Read the model definition and answer for the solid it produces. Units are mm, in the model's axes. Round coordinates to 2 decimals unless told otherwise and drop trailing zeros. Order: outer loops, then holes, each group sorted by start corner. A loop starts at its lowest first (then second) coordinate and runs counter-clockwise, first axis right, second up.
Autodesk Inventor part; units mm, degrees
ref_plane "YZ Plane" through (0, 0, 0) normal (1, 0, 0) x (0, 1, 0)
ref_plane "XZ Plane" through (0, 0, 0) normal (0, 1, 0) x (-1, 0, 0)
ref_plane "XY Plane" through (0, 0, 0) normal (0, 0, 1) x (1, 0, 0)
sketch "스케치1" plane through (0, 0, 0) normal (0, 1, 0) x (-1, 0, 0)
  circle A0 centre (0, 0) radius 15
  circle A1 centre (0, 0) radius 11.5
  line L0 (-14.5237, 3.75) -> (-45, 3.75)
  line L1 (-45, 3.75) -> (-45, -3.75)
  line L2 (-45, -3.75) -> (-14.5237, -3.75)
  line L3 (-14.5237, -3.75) -> (-14.5237, 3.75)
  dimension "d0" = 30
  dimension "d1" = 23
  dimension "d2" = 7.5
  dimension "d3" = 3.75
  dimension "d4" = 45
extrude "돌출1" add sketch "스케치1" along normal blind 1
properties part number "압력센서"
Q1. A cutting plane is placed at A-A, the plane x = 0. Give the vertices of the cut face in (y, z), plus the area to 3 significant figures.
Outcome:
outline: (0, -15) - (1, -15) - (1, -11.5) - (0, -11.5) - close; (0, 11.5) - (1, 11.5) - (1, 15) - (0, 15) - close
area: 7.00 mm2
Q2. Straight lines are drawn through the part: probe 1 along Z at (x, y) = (0, 0.2); probe 2 along X at (y, z) = (0.65, -3); probe 3 along X at (y, z) = (0.35, 1). For each, find the intervals that lie inside material, in ascending order.
Outcome:
probe 1: z = -15 to -11.5, 11.5 to 15
probe 2: x = -14.7 to -11.1, 11.1 to 45
probe 3: x = -14.97 to -11.46, 11.46 to 45
Q3. A flat-ended cylindrical pin translates along its axis: pin 1 (1 mm diameter, centred on x = -1, z = -10.5, fed in from +Y). Find the tip coordinate at first contact, or state that the pin passes through.
Outcome:
pin 1: passes through
Q4. A cutting plane is placed at C-C, the plane y = 0.4. Give the vertices of the cut face in (x, z).
Outcome:
outline: (14.52, -3.75) - (45, -3.75) - (45, 3.75) - (14.52, 3.75) arc R15 ccw (long way) to start; hole circle Ø23 at (0, 0)
Q5. A cutting plane is placed at B-B, the plane z = 0. Give the vertices of the cut face in (x, y), plus the area to 3 significant figures.
Outcome:
outline: (-15, 0) - (-11.5, 0) - (-11.5, 1) - (-15, 1) - close; (11.5, 0) - (45, 0) - (45, 1) - (11.5, 1) - close
area: 37.0 mm2
Q6. A cutting plane is placed at D-D, the plane z = 13. Give the vertices of the cut face in (x, y), plus the area to 3 significant figures.
Outcome:
outline: (-7.48, 0) - (7.48, 0) - (7.48, 1) - (-7.48, 1) - close
area: 15.0 mm2
